Geometry: see drawing. Coordinates: mm, zero at the bounding-box minimum. Coordinates: 2 decimals unless noted, no trailing zeros. Order: outer loops, then holes, each group sorted by start corner. A loop starts at its lowest first (then second) coordinate and runs counter-clockwise, first axis right, second up. Notation, with made-up numbers: (7.25, 37) -> (62.25, 37) arc R26 ccw to (62.25, 74) -> close; hole circle Ø2 at (51.25, 84.5). An arc over 180 degrees is marked (long way). One line per item, written item: value. Start each with the question number.
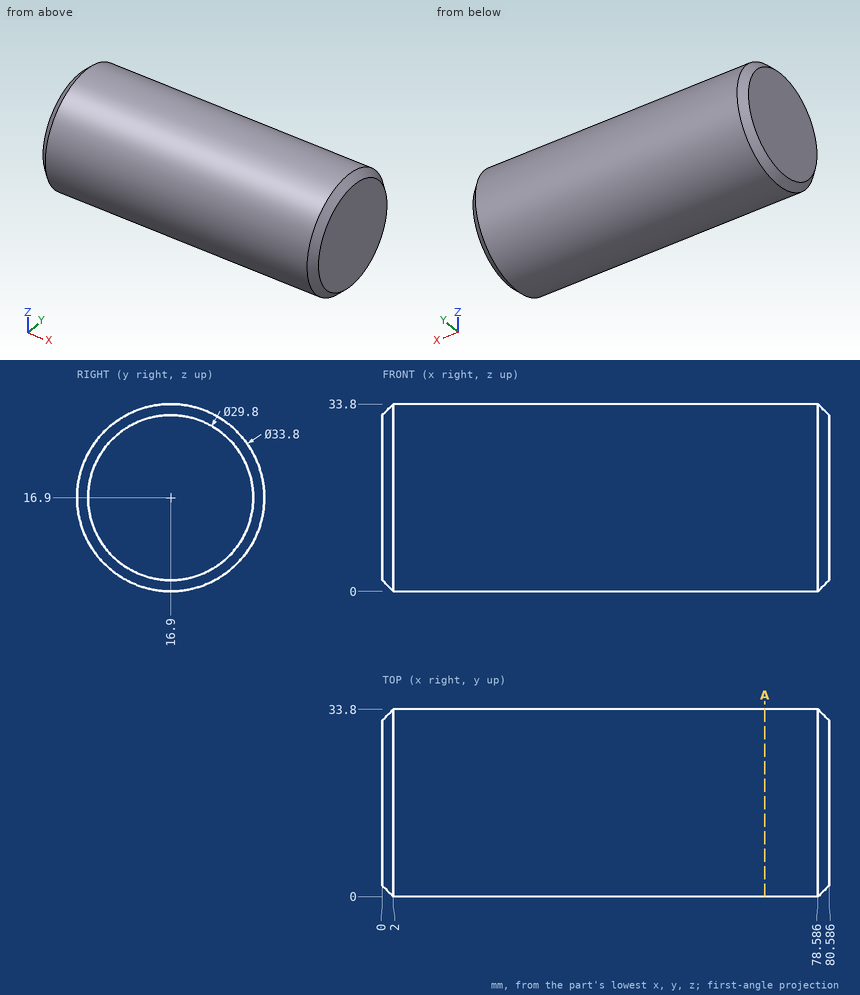
1) Section query A-A, the plane x = 69. Return the cut outline in (y, z), plus the area to 3 significant figures.
2) Ray query, line 1 along Y through (x, z) = (11.5, 17); line 2 along Y through (x, z) = (49.5, 7); line 3 along Z through (x, y) = (48, 27.5). Return the intervals inside material, ascending. Write a range as from..to.
3) Pin query (flat end, axial travel): pin 1 Ø5 at (x, z) = (15, 24.5) entering from +Y; pin 2 Ø1 at (x, y) = (28.5, 27.5) entering from +Z. Return the tip coordinate at first contact, or that it passes through.
Entries:
1. outline: circle Ø33.8 at (16.9, 16.9)
1. area: 897 mm2
2. line 1: y = 0..33.8
2. line 2: y = 3.2..30.6
2. line 3: z = 3.74..30.06
3. pin 1: stops at y = 33.01
3. pin 2: stops at z = 30.45
